Autodesk Inventor part; units mm, degrees
ref_plane "YZ Plane" through (0, 0, 0) normal (1, 0, 0) x (0, 1, 0)
ref_plane "XZ Plane" through (0, 0, 0) normal (0, 1, 0) x (-1, 0, 0)
ref_plane "XY Plane" through (0, 0, 0) normal (0, 0, 1) x (1, 0, 0)
sketch "Sketch1" plane through (0, 0, 0) normal (0, 0, 1) x (1, 0, 0)
  line L0 (0, 0) -> (30.48, 0)
  line L1 (30.48, 0) -> (30.48, 38.1)
  line L2 (30.48, 38.1) -> (0, 38.1)
  line L3 (0, 38.1) -> (0, 0)
  dimension "d0" = 30.48
  dimension "d1" = 38.1
extrude "Extrusion1" add sketch "Sketch1" along normal blind 7.62
sketch "Sketch2" plane through (0, 0, 7.62) normal (0, 0, 1) x (1, 0, 0)
  line L0 (0, 0) -> (30.48, 0)
  line L1 (0, 38.1) -> (0, 0)
  line L2 (30.48, 0) -> (30.48, 38.1)
  line L3 (15.24, 0) -> (15.24, 5.08) construction
  line L4 (15.24, 5.08) -> (7.62, 5.08) construction
  circle A0 centre (7.62, 5.08) radius 2.413
  line L5 (15.24, 5.08) -> (22.86, 5.08) construction
  circle A1 centre (22.86, 5.08) radius 2.413
  dimension "d4" = 5.08
  dimension "d5" = 7.62
  dimension "d6" = 4.826
extrude "Extrusion2" cut sketch "Sketch2" against normal blind 7.62
sketch "Sketch3" plane through (0, 0, 7.62) normal (0, 0, 1) x (1, 0, 0)
  line L0 (0, 38.1) -> (0, 0)
  line L1 (30.48, 38.1) -> (0, 38.1)
  line L2 (30.48, 0) -> (30.48, 38.1)
  line L3 (15.24, 38.1) -> (15.24, 24.13) construction
  circle A0 centre (15.24, 24.13) radius 2.413
  dimension "d9" = 13.97
  dimension "d10" = 4.826
extrude "Extrusion3" cut sketch "Sketch3" against normal blind 7.62
sketch "Sketch4" plane through (0, 0, 7.62) normal (0, 0, 1) x (1, 0, 0)
  line L0 (0, 38.1) -> (0, 0)
  line L1 (30.48, 38.1) -> (0, 38.1)
  line L2 (30.48, 0) -> (30.48, 38.1)
  circle A0 centre (15.24, 24.13) radius 2.413
  line L3 (15.24, 24.13) -> (15.24, 38.1) construction
  arc A1 (9.7407, 27.305) -> (19.6524, 28.6965) centre (15.24, 24.13) ccw construction
  arc A2 (5.5613, 29.718) -> (23.0058, 32.1671) centre (15.24, 24.13) ccw construction
  line L4 (15.24, 24.13) -> (9.7407, 27.305) construction
  line L5 (15.24, 24.13) -> (25.654, 24.13) construction
  line L6 (15.24, 24.13) -> (20.7393, 27.305) construction
  line L7 (15.24, 24.13) -> (25.654, 24.13) construction
  line L8 (9.7407, 27.305) -> (5.5613, 29.718) construction
  line L9 (20.7393, 27.305) -> (24.9187, 29.718) construction
  arc A3 (7.4742, 32.1671) -> (10.8276, 28.6965) centre (9.1509, 30.4318) ccw
  arc A4 (19.6524, 28.6965) -> (23.0058, 32.1671) centre (21.3291, 30.4318) ccw
  arc A5 (7.4742, 32.1671) -> (5.5613, 29.718) centre (15.24, 24.13) ccw construction
  arc A6 (10.8276, 28.6965) -> (9.7407, 27.305) centre (15.24, 24.13) ccw construction
  arc A7 (19.6524, 28.6965) -> (10.8276, 28.6965) centre (15.24, 24.13) ccw
  arc A8 (23.0058, 32.1671) -> (7.4742, 32.1671) centre (15.24, 24.13) ccw
  arc A9 (23.0058, 32.1671) -> (19.6524, 28.6965) centre (21.3291, 30.4318) ccw construction
  arc A10 (10.8276, 28.6965) -> (7.4742, 32.1671) centre (9.1509, 30.4318) ccw construction
  dimension "d13" = 12.7
  dimension "d14" = 22.352
  dimension "d15" = 150
  dimension "d16" = 30
  dimension "d17" = 4.826
  dimension "d18" = 4.826
extrude "Extrusion4" cut sketch "Sketch4" against normal through all contours A8 A4 A7 A3
properties part number "arm_camera_adapter"
Geometry: final body of the model. Coordinates: model frame, mm. A direction names the side the tool comes from. Coordinates: 2 decimals unless noted, no trailing zeros. Order: outer loops, then holes, each group sorted by start corner. A loop starts at its lowest first (then second) coordinate and runs counter-clockwise, first axis right, second up. Notation, with made-up numbers: (76.25, -8.75) -> (126.25, -8.75) arc R20 cw to (126.25, 6.25) -> close; hole circle Ø11 at (-26.5, -30.5). An arc over 180 degrees is marked (long way). Write item = value, one per line.
(1) Cut plane A-A on y = 5.08. Return loops of the section in (x, z).
Solved:
outline = (0, 0) -> (5.21, 0) -> (5.21, 7.62) -> (0, 7.62) -> close; (10.03, 0) -> (20.45, 0) -> (20.45, 7.62) -> (10.03, 7.62) -> close; (25.27, 0) -> (30.48, 0) -> (30.48, 7.62) -> (25.27, 7.62) -> close
(2) Cut plane B-B on z = 3. Return loops of the section in (x, y).
Solved:
outline = (0, 0) -> (30.48, 0) -> (30.48, 38.1) -> (0, 38.1) -> close; hole circle Ø4.83 at (7.62, 5.08); hole (7.47, 32.17) arc R2.41 ccw to (10.83, 28.7) arc R6.35 cw to (19.65, 28.7) arc R2.41 ccw to (23.01, 32.17) arc R11.18 ccw to start; hole circle Ø4.83 at (15.24, 24.13); hole circle Ø4.83 at (22.86, 5.08)
(3) Cut plane C-C on x = 24.5. Return loops of the section in (y, z).
Solved:
outline = (0, 0) -> (3.31, 0) -> (3.31, 7.62) -> (0, 7.62) -> close; (6.85, 0) -> (38.1, 0) -> (38.1, 7.62) -> (6.85, 7.62) -> close
(4) Access query for faces 5 (the cylindrical face through (15.31, 30.48, 3.86)), 6 (the flat face through (15, 19, 7.62)). Directions: +Z, -Z, +X, -X, +Y, -Y. A direction counts if a zero-diameter tool reaches every point of the face in a straight line with its end or side. Return the directions, or none.
Solved:
face_5 = +Z, -Z
face_6 = +Z, +X, -X, +Y, -Y
(5) Pull-direction query (X, two-part tool) for faces 1 (the flat face through (0, 19, 4)), 2 (the cylindrical face through (7.38, 28.79, 3.86)), 3 (the flat face through (15, 19, 0)), 4 (the flat face through (30.48, 19, 4)); classes: pulls with the +X half, pulls with the -X half, needs draft (parallel to the pull), parting line crosses it, or undercut.
Solved:
face_1 = pulls with the -X half
face_2 = undercut
face_3 = needs draft
face_4 = pulls with the +X half
(6) Pin query (flat end, axial travel): pin 1 Ø10 at (x, y) = (3, 5) entering from -Z; pin 2 Ø3 at (x, y) = (15.24, 24.13) entering from +Z. Return the tip coordinate at first contact, or that it passes through.
Solved:
pin_1 = 0
pin_2 = through
(7) Cut plane D-D on y = 24.13. Return loops of the section in (x, z).
Solved:
outline = (0, 0) -> (12.83, 0) -> (12.83, 7.62) -> (0, 7.62) -> close; (17.65, 0) -> (30.48, 0) -> (30.48, 7.62) -> (17.65, 7.62) -> close
(8) Line query: line 1 (Y direction, x = 22.86, z = 5.25); line 2 (Y direction, x = 15, z = 5.75); line 3 (Y direction, x = 24, z = 2). Output: solid intervals per line, ascending.
Solved:
line_1 = 0 to 2.67, 7.49 to 28.57, 32.31 to 38.1
line_2 = 0 to 21.73, 26.53 to 30.48, 35.3 to 38.1
line_3 = 0 to 2.95, 7.21 to 38.1
